Job drawing, mm, ordinate dimensions from the low corner. One solid piece. A direction names the side the tool comes from. Round coordinates to 2 decimals unless told otherwise and drop trailing zeros. Loops run counter-clockwise (first coordinate to the right, second up) from the corner with the lowest first, then second, coordinate; pieces in that order, holes last. Notation, with made-up numbers: M 63.5,31 L 82.5,31 A18 cw 82.5,43 Z; hole C 72,-34.5 d2. An arc over 180 degrees is marked long. Put each result on its own line as item: value. Start each with the question number.
1) Probe line 1 along Z through (x, y) = (4, 3.75) (3 decimals); line 2 along X through (y, z) = (6.5, 1); line 3 along Y through (x, z) = (24.5, 23). List the from-to ranges inside material, lowest first.
2) Slice it at B-B on y = 4.5. Give the cut face in (x, z) (1 decimal), then the cut area to 3 significant figures.
3) Which spindle directions (+Z, -Z, +X, -X, +Y, -Y) get a long thin tool onto all of the face, cutting with end or side? Do the marked faces 1 and 2. Say none if no direction does.
4) Slice it at C-C on z = 11.75. Give the cut face in (x, y).
5) Pull direction X, two halves, no side cores. Call the marked faces 3, 4 and 5: +X half, -X half, draft (parallel to the pull), parting line (faces both ways), or undercut.
6) Drop flat-ended pins along their axis: pin 1 Ø3.5 at (x, z) = (4, 20.825) entering from -Y; pin 2 Ø13 at (x, z) = (19.5, 10) entering from +Y. Give the stop position or say it passes through.
7) Slice it at A-A on x = 4. Give the cut face in (y, z) (3 decimals), then the cut area to 3 significant figures.
8) Slice it at D-D on x = 22. Give the cut face in (y, z).
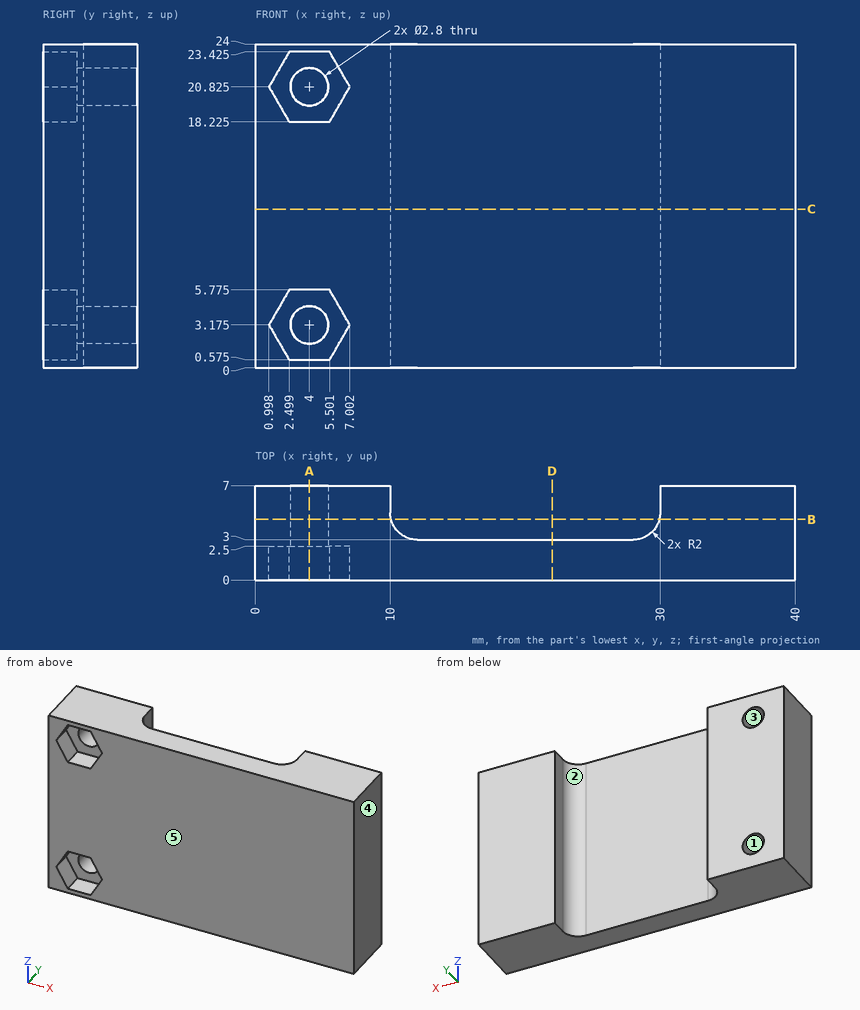
Recorded:
1. line 1: z = 0 to 1.775, 4.575 to 19.425, 22.225 to 24
1. line 2: x = 0 to 10, 30 to 40
1. line 3: y = 0 to 3
2. outline: M 0,0 L 10.1,0 L 10.1,24 L 0,24 Z; M 29.9,0 L 40,0 L 40,24 L 29.9,24 Z; hole C 4,3.2 d2.8; hole C 4,20.8 d2.8
2. area: 471 mm2
3. face 1: +Y, -Y
3. face 2: +Z, -Z, +Y
4. outline: M 0,0 L 40,0 L 40,7 L 30,7 L 30,5 A2 cw 28,3 L 12,3 A2 cw 10,5 L 10,7 L 0,7 Z
5. face 3: undercut
5. face 4: +X half
5. face 5: draft
6. pin 1: stops at y = 2.5
6. pin 2: stops at y = 3
7. outline: M 0,0 L 7,0 L 7,1.775 L 2.5,1.775 L 2.5,0.575 L 0,0.575 Z; M 0,5.775 L 2.5,5.775 L 2.5,4.575 L 7,4.575 L 7,19.425 L 2.5,19.425 L 2.5,18.225 L 0,18.225 Z; M 0,23.425 L 2.5,23.425 L 2.5,22.225 L 7,22.225 L 7,24 L 0,24 Z
7. area: 117 mm2
8. outline: M 0,0 L 3,0 L 3,24 L 0,24 Z
